The model under review builds one solid part; all positions refer to its coordinate system, in mm. Face numbers are marked on the shaded views. A direction names the side the tool comes from. Round coordinates to 2 decimals unless told otherwise and drop trailing zeros. Order: outer loops, then holes, each group sorted by start corner. A loop starts at its lowest first (then second) coordinate and runs counter-clockwise, first axis right, second up. Notation, with made-up numbers: (51.5, 30.5) -> (99.5, 30.5) arc R27 ccw to (99.5, 61.5) -> close; hole circle Ø1 at (23.25, 7). An arc over 180 degrees is marked (long way). Use a Markdown table: item, result. Add a question column.
```python
from build123d import *

# Parameters (mm, degrees)
SKETCH2_W           = 20.32
SKETCH2_H           = 17.78
SKETCH2_R           = 1.5
BOSS_EXTRUDE1_DEPTH = 2
SKETCH3_R           = 2.9
BOSS_EXTRUDE2_DEPTH = 2.2
SKETCH4_R           = 2.15
CUT_EXTRUDE1_DEPTH  = 1
FILLET2_R           = 0.5


with BuildPart() as part:
    # Sketch2 → Boss-Extrude1 (new body)
    with BuildSketch(Plane(origin=(0, 0, 0), x_dir=(1, 0, 0), z_dir=(0, 1, 0))):
        Rectangle(SKETCH2_W, SKETCH2_H)
        with Locations(Location((7.62, 6.35, 0), (0, 0, 270))):
            Circle(SKETCH2_R, mode=Mode.SUBTRACT)
        with Locations(Location((-7.62, -1.27, 0), (0, 0, 270))):
            Circle(SKETCH2_R, mode=Mode.SUBTRACT)
    extrude(amount=BOSS_EXTRUDE1_DEPTH)

    # Sketch3 → Boss-Extrude2 (add)
    with BuildSketch(Plane(origin=(0, 2, 0), x_dir=(1, 0, 0), z_dir=(0, 1, 0))):
        with Locations(Location((0, 2.54, 0), (0, 0, 270))):
            Circle(SKETCH3_R)
    extrude(amount=BOSS_EXTRUDE2_DEPTH)

    # Sketch4 → Cut-Extrude1 (cut)
    with BuildSketch(Plane(origin=(0, 4.2, 0), x_dir=(1, 0, 0), z_dir=(0, 1, 0))):
        with Locations(Location((0, 2.54, 0), (0, 0, 270))):
            Circle(SKETCH4_R)
    extrude(amount=-CUT_EXTRUDE1_DEPTH, mode=Mode.SUBTRACT)

    # Fillet2
    fillet2_edges = [part.edges().sort_by_distance(p)[0] for p in [
        (0, 3.2, -4.69),
    ]]
    fillet(fillet2_edges, radius=FILLET2_R)


solid = part.part
```
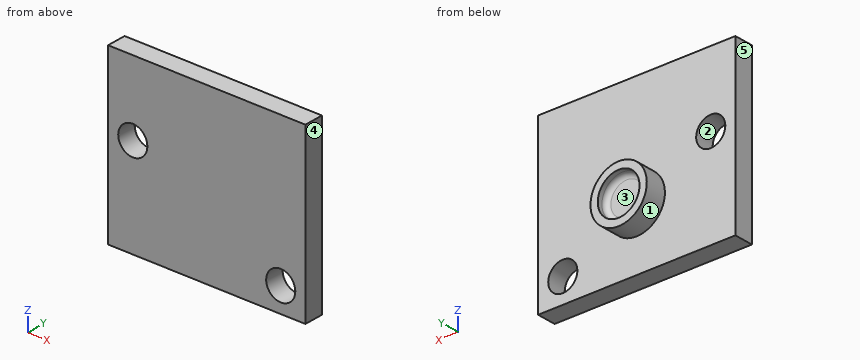
Q1. Add section C-C (y = 0.7). Write out the cut boundary in (x, z), then the cut area to 3 significant figures.
Q2. Wall thickness on line 1 (X direction, y = 4, z = -2.5); line 2 (X direction, y = 0.75, z = -6.35); line 3 (Y direction, x = -2.5, z = -7): over which ranges is each line inside the solid? List them lowest first. Write a range as [from, to].
Q3. Mouldability with a two-part tool opening along X and no side actions: class the marked faces 3, 4 and 5 as pulls with the +X half, pulls with the -X half, needs draft (parallel to the pull), parting line crosses it, or undercut.
Q4. Add section D-D (x = 0). Write out the cut boundary in (y, z).
Q5. Add section B-B (x = -7.62). Write out the cut boundary in (y, z).
Q6. Machinability: for the marked faces 1 and 2, which of the approach directions +Z, -Z, +X, -X, +Y, -Y give a long, thin tool a straight path to every point of the face, cutting with its end or side? Answer none if there is none.
Q7. Add section A-A (z = -6.35). Write out the cut boundary in (x, y).
Q8. Insertion check: pin 1 (5 mm diameter, centred on x = 7.62, z = -6.35, fed in from +Y); pin 2 (1 mm diameter, centred on x = -0.5, z = -3, fed in from +Y). Each pin has a flat end and moves straight along its axis. Give the tip position at first contact, or say it passes through.
Report:
| question | item | result |
|---|---|---|
| 1 | outline | (-10.16, -8.89) -> (10.16, -8.89) -> (10.16, 8.89) -> (-10.16, 8.89) -> close; hole circle Ø3 at (-7.62, 1.27); hole circle Ø3 at (7.62, -6.35) |
| 1 | area | 347 mm² |
| 2 | line 1 | x = [-2.9, -2.15], [2.15, 2.9] |
| 2 | line 2 | x = [-10.16, 6.12], [9.12, 10.16] |
| 2 | line 3 | y = [0, 2] |
| 3 | face 3 | undercut |
| 3 | face 4 | pulls with the +X half |
| 3 | face 5 | pulls with the -X half |
| 4 | outline | (0, -8.89) -> (2, -8.89) -> (2, -5.44) -> (4.2, -5.44) -> (4.2, -4.69) -> (3.7, -4.69) arc R0.5 cw to (3.2, -4.19) -> (3.2, -0.89) arc R0.5 cw to (3.7, -0.39) -> (4.2, -0.39) -> (4.2, 0.36) -> (2, 0.36) -> (2, 8.89) -> (0, 8.89) -> close |
| 5 | outline | (0, -8.89) -> (2, -8.89) -> (2, -0.23) -> (0, -0.23) -> close; (0, 2.77) -> (2, 2.77) -> (2, 8.89) -> (0, 8.89) -> close |
| 6 | face 1 | +Y |
| 6 | face 2 | +Y, -Y |
| 7 | outline | (-10.16, 0) -> (6.12, 0) -> (6.12, 2) -> (-10.16, 2) -> close; (9.12, 0) -> (10.16, 0) -> (10.16, 2) -> (9.12, 2) -> close |
| 8 | pin 1 | stops at y = 2 |
| 8 | pin 2 | stops at y = 3.2 |
